Input: dimensioned drawing with shaded views. Units: mm. Origin: part minimum x, y, z. A direction names the side the tool comes from. Give positions to 0.01 mm unless a question says otherwise; leave off trailing zeros. Loops run counter-clockwise (first coordinate to the right, second up) from the corner with the lowest first, then second, coordinate; pieces in that order, holes last. Notation, with made-up numbers: (37.25, 22.5) -> (47.25, 22.5) arc R23 cw to (47.25, 50.5) -> close; hole circle Ø11 at (-16, 63). An arc over 180 degrees is marked (long way). Answer as a JSON object with one key per item and string values.
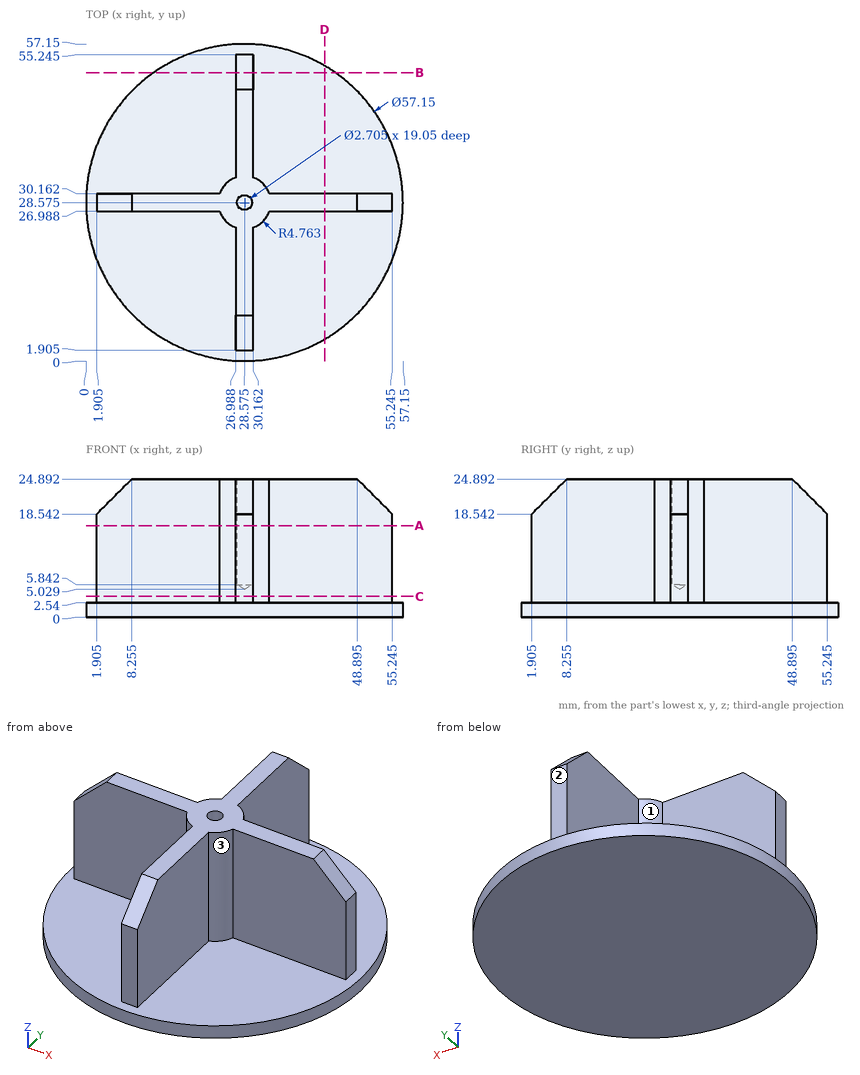
Q1. Ray query, line 1 along Y through (x, z) = (43, 14.5); line 2 along Z through (x, y) = (12, 42.5). Return the intervals inside material, ascending.
Evaluation:
{"line 1": "y = 26.99 to 30.16", "line 2": "z = 0 to 2.54"}
Q2. Section D-D, the plane x = 43. Return the cut outline in (y, z), then the cut area to 3 significant figures.
Evaluation:
{"outline": "(3.91, 0) -> (53.24, 0) -> (53.24, 2.54) -> (30.16, 2.54) -> (30.16, 24.89) -> (26.99, 24.89) -> (26.99, 2.54) -> (3.91, 2.54) -> close", "area": "196 mm2"}
Q3. Section B-B, the plane y = 52. Return the cut outline in (x, z), then the cut area to 3 significant figures.
Evaluation:
{"outline": "(12.21, 0) -> (44.94, 0) -> (44.94, 2.54) -> (30.16, 2.54) -> (30.16, 21.79) -> (26.99, 21.79) -> (26.99, 2.54) -> (12.21, 2.54) -> close", "area": "144 mm2"}
Q4. Access query for the marked faces 1, 2 and 3. Directions: +Z, -Z, +X, -X, +Y, -Y. A direction counts if a zero-diameter tool reaches every point of the face in a straight line with its end or side. Return the directions, or none.
Evaluation:
{"face 1": "+Z, -X, +Y", "face 2": "+Z, +X, -X, +Y", "face 3": "+Z, +X, -Y"}
Q5. Section A-A, the plane z = 16.5. Return the cut outline in (x, y) (1 decimal), then the cut area to 3 significant figures.
Evaluation:
{"outline": "(1.9, 27) -> (24.1, 27) arc R4.8 ccw to (27, 24.1) -> (27, 1.9) -> (30.2, 1.9) -> (30.2, 24.1) arc R4.8 ccw to (33.1, 27) -> (55.2, 27) -> (55.2, 30.2) -> (33.1, 30.2) arc R4.8 ccw to (30.2, 33.1) -> (30.2, 55.2) -> (27, 55.2) -> (27, 33.1) arc R4.8 ccw to (24.1, 30.2) -> (1.9, 30.2) -> close; hole circle Ø2.7 at (28.6, 28.6)", "area": "345 mm2"}
Q6. Pin query (flat end, axial travel): pin 1 (1.5 mm diameter, centred on x = 29, z = 6.5, fed in from +Y) (1 decimal); pin 2 (6.5 mm diameter, centred on x = 14.5, z = 13.5, fed in from +Y); pin 3 (11 mm diameter, centred on y = 42, z = 16, fed in from +X). Return the tip coordinate at first contact, or that it passes through.
Evaluation:
{"pin 1": "stops at y = 55.2", "pin 2": "stops at y = 30.16", "pin 3": "stops at x = 30.16"}
Q7. Section C-C, the plane z = 3.75. Return the cut outline in (x, y) (1 decimal).
Evaluation:
{"outline": "(1.9, 27) -> (24.1, 27) arc R4.8 ccw to (27, 24.1) -> (27, 1.9) -> (30.2, 1.9) -> (30.2, 24.1) arc R4.8 ccw to (33.1, 27) -> (55.2, 27) -> (55.2, 30.2) -> (33.1, 30.2) arc R4.8 ccw to (30.2, 33.1) -> (30.2, 55.2) -> (27, 55.2) -> (27, 33.1) arc R4.8 ccw to (24.1, 30.2) -> (1.9, 30.2) -> close"}
